Autodesk Inventor part; units mm, degrees
ref_plane "YZ Plane" through (0, 0, 0) normal (1, 0, 0) x (0, 1, 0)
ref_plane "XZ Plane" through (0, 0, 0) normal (0, 1, 0) x (-1, 0, 0)
ref_plane "XY Plane" through (0, 0, 0) normal (0, 0, 1) x (1, 0, 0)
sketch "スケッチ1" plane through (0, 0, 0) normal (0, 0, 1) x (1, 0, 0)
  line L0 (-28, -31.5) -> (28, -31.5) construction
  line L1 (28, -31.5) -> (28, 31.5) construction
  line L2 (28, 31.5) -> (-28, 31.5) construction
  line L3 (-28, 31.5) -> (-28, -31.5) construction
  line L4 (-28, -31.5) -> (28, 31.5) construction
  line L5 (28, -31.5) -> (-28, 31.5) construction
  line L6 (-28, 10.6) -> (-28, 31.5)
  line L7 (-28, 31.5) -> (28, 31.5)
  line L8 (28, 31.5) -> (28, 10.6)
  line L9 (-28, -10.6) -> (-28, -31.5)
  line L10 (-28, -31.5) -> (28, -31.5)
  line L11 (28, -31.5) -> (28, -10.6)
  line L12 (-28, 8.5) -> (-33, 8.5)
  line L13 (-33, 8.5) -> (-33, -8.5)
  line L14 (-33, -8.5) -> (-28, -8.5)
  line L15 (28, 8.5) -> (33, 8.5)
  line L16 (33, 8.5) -> (33, -8.5)
  line L17 (33, -8.5) -> (28, -8.5)
  line L18 (0, 0) -> (0, 31.5) construction
  line L19 (0, 0) -> (28, 0) construction
  arc A0 (-28, 8.5) -> (-28, 10.6) centre (-28, 9.55) ccw
  arc A1 (-28, -10.6) -> (-28, -8.5) centre (-28, -9.55) ccw
  arc A2 (28, 10.6) -> (28, 8.5) centre (28, 9.55) ccw
  arc A3 (28, -8.5) -> (28, -10.6) centre (28, -9.55) ccw
  dimension "d45" = 63
  dimension "d73" = 56
  dimension "d74" = 1.05
  dimension "d75" = 5
  dimension "d76" = 23
extrude "押し出し1" add sketch "スケッチ1" along normal blind 5
sketch "スケッチ2" plane through (0, 0, 5) normal (0, 0, 1) x (1, 0, 0)
  line L0 (-28, 31.5) -> (-28, 10.6)
  line L1 (28, 10.6) -> (28, 31.5)
  line L2 (-50.9845, 57.5344) -> (-28, 57.5344)
  line L3 (-28, 57.5344) -> (-28, -57.37)
  line L4 (-28, -57.37) -> (-50.9845, -57.37)
  line L5 (-50.9845, -57.37) -> (-50.9845, 57.5344)
  line L6 (28, 64.7229) -> (65.0267, 64.7229)
  line L7 (65.0267, 64.7229) -> (65.0267, -57.37)
  line L8 (65.0267, -57.37) -> (28, -57.37)
  line L9 (28, -57.37) -> (28, 64.7229)
  point P0 (0, 0)
extrude "押し出し2" cut sketch "スケッチ2" against normal blind 2.5
equation "\"d45\" = d1"
equation "\"d76\" = d20 + d23"
properties part number "コックピット_2_サブフレーム_4" material "アセタール樹脂、黒"
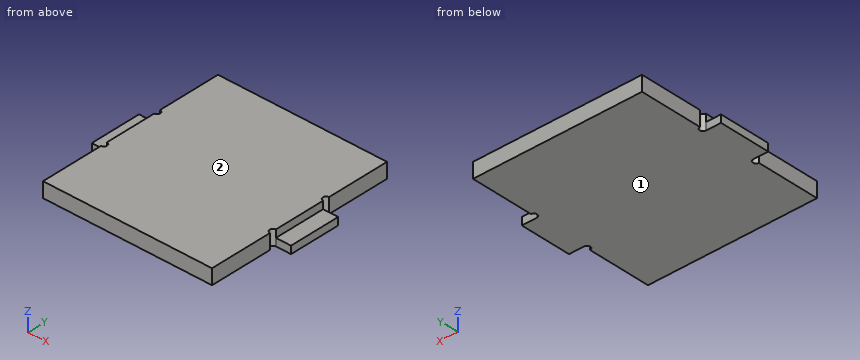
Read the model definition and answer for the solid it produces. Units are mm, in the model's axes. Face numbers are marked on the shaded views. Round coordinates to 2 decimals unless told otherwise and drop trailing zeros. Write each loop counter-clockwise with the first axis right and the second up, starting at its lowest first coordinate (ties: lowest second). Pieces come first, ordered by that corner, then holes. Notation, with made-up numbers: (-6.5, 61) - (15.5, 61) arc R14 ccw to (15.5, 65) - close; hole circle Ø10 at (16.5, 80). An arc over 180 degrees is marked (long way). One line per question, with ' | ' between items. Start each with the question number.
1. For a pull along Z with two mould halves and no side action, classify the marked faces 1 and 2 as +Z half, -Z half, draft (parallel to the pull), parting line (faces both ways), or undercut.
2. Each of these flat-tipped pins is pushed along its axis until it touches: pin 1 (0.8 mm diameter, centred on y = 3, z = 3.5, fed in from -X); pin 2 (0.8 mm diameter, centred on x = 30, z = 1, fed in from -Y); pin 3 (1.2 mm diameter, centred on y = 1, z = 4, fed in from +X). Where does it stop, or does it pass through?
3. Section A-A (y = -1) is taken. Determine the outline of the cut face in (x, z), and give its area (3 significant figures).
4. Section C-C (y = 9.55) is taken. Determine the outline of the cut face in (x, z).
5. Find the intervals of material crossed by probe 1 along X at (y, z) = (2, 2.65); probe 2 along X at (y, z) = (10.5, 2.45), in increasing order. Write a range as [from, to].
6. Section B-B (y = -20.5) is taken. Determine the outline of the cut face in (x, z), and give its area (3 significant figures).
Filled in:
1) face 1: -Z half | face 2: +Z half
2) pin 1: x = -28 | pin 2: y = -8.5 | pin 3: x = 28
3) outline: (-33, 0) - (33, 0) - (33, 2.5) - (28, 2.5) - (28, 5) - (-28, 5) - (-28, 2.5) - (-33, 2.5) - close | area: 305 mm²
4) outline: (-26.95, 0) - (26.95, 0) - (26.95, 5) - (-26.95, 5) - close
5) probe 1: [-28, 28] | probe 2: [-27.55, 27.55]
6) outline: (-28, 0) - (28, 0) - (28, 5) - (-28, 5) - close | area: 280 mm²
